Input: part model. Units: mm. Frame: model coordinates. A direction names the side the tool comes from. Round coordinates to 2 decimals unless told otherwise and drop trailing zeros. Order: outer loops, then holes, each group sorted by start corner. A loop starts at its lowest first (then second) coordinate and runs counter-clockwise, first axis right, second up. Notation, with made-up numbers: (-36, 25) - (-4, 25) arc R14 ccw to (-4, 52) - close; hole circle Ø9 at (-5.5, 15). An arc over 180 degrees is marked (long way). One line per item, written item: value. Start each with the question number.
from build123d import *

# Parameters (mm, degrees)
SKICA1_R                 = 4
SKICA1_W                 = 1.7
SKICA1_H                 = 7.8
SKICA1_R_2               = 1.5
P_IDAT_VYSUNUT_M3_DEPTH  = 1.4
SKICA3_R                 = 3.986213299
ODEBRAT_VYSUNUT_M1_DEPTH = 0.9
SKICA7_W                 = 1.7
SKICA7_H                 = 7.8
P_IDAT_VYSUNUT_M5_DEPTH  = 1.4


with BuildPart() as part:
    # Skica1 → P_idat vysunut_m3 (new body)
    # profile 1 of 3: a face of its own
    with BuildSketch(Plane.XY):
        with BuildLine():
            ThreePointArc((-11.45, -6.25), (-11.803553391, -6.103553391), (-11.95, -5.75))
            Line((-11.95, -5.75), (-11.95, 3.25))
            ThreePointArc((-11.95, 3.25), (-11.071320344, 5.371320344), (-8.95, 6.25))
            Line((-8.95, 6.25), (8.95, 6.25))
            ThreePointArc((8.95, 6.25), (11.071320344, 5.371320344), (11.95, 3.25))
            Line((11.95, 3.25), (11.95, -5.75))
            ThreePointArc((11.95, -5.75), (11.803553391, -6.103553391), (11.45, -6.25))
            Line((11.45, -6.25), (-11.45, -6.25))
        make_face()
        with Locations((-6, 0.95)):
            Circle(SKICA1_R, mode=Mode.SUBTRACT)
        with Locations((6, 0.95)):
            Circle(SKICA1_R, mode=Mode.SUBTRACT)
        Rectangle(SKICA1_W, SKICA1_H, mode=Mode.SUBTRACT)
    # profile 2 of 3: a face of its own
    with BuildSketch(Plane.XY):
        with Locations((-6, 0.95)):
            Circle(SKICA1_R)
        with Locations((-6, 0.95)):
            Circle(SKICA1_R_2, mode=Mode.SUBTRACT)
    # profile 3 of 3: a face of its own
    with BuildSketch(Plane.XY):
        with Locations((6, 0.95)):
            Circle(SKICA1_R)
        with Locations((6, 0.95)):
            Circle(SKICA1_R_2, mode=Mode.SUBTRACT)
    extrude(amount=P_IDAT_VYSUNUT_M3_DEPTH)

    # Skica3 → Odebrat vysunut_m1 (cut)
    with BuildSketch(Plane(origin=(0, 0, 0), x_dir=(-1, 0, 0), z_dir=(0, 0, -1))):
        with Locations((-6, 0.95)):
            Circle(SKICA3_R)
        with Locations((6, 0.95)):
            Circle(SKICA3_R)
    extrude(amount=-ODEBRAT_VYSUNUT_M1_DEPTH, mode=Mode.SUBTRACT)

    # Skica7 → P_idat vysunut_m5 (add)
    with BuildSketch(Plane(origin=(0, 0, 0), x_dir=(-1, 0, 0), z_dir=(0, 0, -1))):
        Rectangle(SKICA7_W, SKICA7_H)
    extrude(amount=-P_IDAT_VYSUNUT_M5_DEPTH)


solid = part.part
Item 1: Section query C-C on z = 0.4. Return loops of the section in (x, y).
Item 2: Section query A-A on y = 0.95. Return loops of the section in (x, z).
Item 3: Section query D-D on x = -8.5. Return loops of the section in (y, z).
Item 4: Pull-direction query (X, two-part tool) for faces 3 (the face through (0, -6.25, 1)), 4 (the face through (-7.5, 1, 1.1)), 5 (the face through (-11.95, -1, 1)); classes: released by +X, released by -X, zero draft, split by the parting line, or undercut.
Item 5: First-contact query: pin 1 Ø3.5 at (x, y) = (-6, 0.95) entering from -Z. Flat tip, straight axial feed; report the tip coordinate or a pass-through.
Item 6: Reachability of faces 1 (the face through (4.89, 1.96, 1.15)), 2 (the face through (3.857, 4.311, 0.444)) from +Z, -Z, +X, -X, +Y, -Y: full face, straight path, thin tool, end or side. Return the list, or none.
Item 7: Section query B-B on x = 6. Return loops of the section in (y, z).
Item 8: Line query: L1, parallel to X at y = 0.95, z = 1.3; L2, parallel to Y at x = -6, z = 1.3; L3, parallel to Y at x = 6, z = 0.1. Output: solid intervals per line, ascending.
Geometry results:
1. outline: (-11.95, -5.75) arc R0.5 ccw to (-11.45, -6.25) - (11.45, -6.25) arc R0.5 ccw to (11.95, -5.75) - (11.95, 3.25) arc R3 ccw to (8.95, 6.25) - (-8.95, 6.25) arc R3 ccw to (-11.95, 3.25) - close; hole circle Ø7.97 at (-6, 0.95); hole circle Ø7.97 at (6, 0.95)
2. outline: (-11.95, 0) - (-9.99, 0) - (-9.99, 0.9) - (-7.5, 0.9) - (-7.5, 1.4) - (-11.95, 1.4) - close; (-4.5, 0.9) - (-2.01, 0.9) - (-2.01, 0) - (2.01, 0) - (2.01, 0.9) - (4.5, 0.9) - (4.5, 1.4) - (-4.5, 1.4) - close; (7.5, 0.9) - (9.99, 0.9) - (9.99, 0) - (11.95, 0) - (11.95, 1.4) - (7.5, 1.4) - close
3. outline: (-6.25, 0) - (-2.15, 0) - (-2.15, 0.9) - (4.05, 0.9) - (4.05, 0) - (6.25, 0) - (6.25, 1.4) - (-6.25, 1.4) - close
4. face 3: zero draft
4. face 4: undercut
4. face 5: released by -X
5. pin 1: stops at z = 0.9
6. face 1: +Z, -Z
6. face 2: -Z
7. outline: (-6.25, 0) - (-3.04, 0) - (-3.04, 0.9) - (-0.55, 0.9) - (-0.55, 1.4) - (-6.25, 1.4) - close; (2.45, 0.9) - (4.94, 0.9) - (4.94, 0) - (6.25, 0) - (6.25, 1.4) - (2.45, 1.4) - close
8. L1: x = -11.95 to -7.5, -4.5 to 4.5, 7.5 to 11.95
8. L2: y = -6.25 to -0.55, 2.45 to 6.25
8. L3: y = -6.25 to -3.04, 4.94 to 6.25
